For this review, take the finished solid that the model builds, in its own axes (mm). Give positions to 0.01 mm unless a question says otherwise; leave off trailing zeros. Order: outer loops, then holes, each group sorted by start corner. A loop starts at its lowest first (then second) coordinate and runs counter-clockwise, first axis right, second up.
from build123d import *

# Parameters (mm, degrees)
CROQUIS1_W              = 56
CROQUIS1_H              = 55
SALIENTE_EXTRUIR1_DEPTH = 3
CROQUIS2_R              = 1.3
CORTAR_EXTRUIR1_DEPTH   = 4
CROQUIS3_R              = 6.3
CROQUIS3_R_2            = 1.25
CORTAR_EXTRUIR2_DEPTH   = 4


with BuildPart() as part:
    # Croquis1 → Saliente-Extruir1 (new body)
    with BuildSketch(Plane.XY):
        with Locations((1.5, 0)):
            Rectangle(CROQUIS1_W, CROQUIS1_H)
    extrude(amount=SALIENTE_EXTRUIR1_DEPTH)

    # Croquis2 → Cortar-Extruir1 (cut)
    with BuildSketch(Plane.XY.offset(3)):
        with Locations((25.5, 23.528824725)):
            Circle(CROQUIS2_R)
        with Locations((19.5, 23.528824725)):
            Circle(CROQUIS2_R)
        with Locations((-22.5, 23.528824725)):
            Circle(CROQUIS2_R)
        with Locations((-16.5, 23.528824725)):
            Circle(CROQUIS2_R)
        with Locations((24.5, -14.75)):
            Circle(CROQUIS2_R)
    extrude(amount=-CORTAR_EXTRUIR1_DEPTH, mode=Mode.SUBTRACT)

    # Croquis3 → Cortar-Extruir2 (cut)
    with BuildSketch(Plane(origin=(0, 0, 0), x_dir=(-1, 0, 0), z_dir=(0, 0, -1))):
        with Locations((7, 8.5)):
            Circle(CROQUIS3_R)
        with Locations((20.6, 8.5)):
            Circle(CROQUIS3_R_2)
        with Locations((-6.1, 8.5)):
            Circle(CROQUIS3_R_2)
    extrude(amount=-CORTAR_EXTRUIR2_DEPTH, mode=Mode.SUBTRACT)


solid = part.part
1) Clearance check with a flat-ended pin moving along its axis: pin 1 (1.6 mm diameter, centred on x = -22.5, y = 23.53, fed in from +Z). State where the tip first meets the part, or that it passes through.
Answer sheet:
pin 1: passes through
2) Draft analysis for pull direction Y (two halves, no side actions). For faces 1 (the face through (-23.458, 24.407, 1.521)), 2 (the face through (1, 27.5, 1)), 3 (the face through (1, -27.5, 1)), 4 (the face through (1, 0, 0)), state which applies: +Y half, -Y half, draft (parallel to the pull), parting line (faces both ways), or undercut.
Answer sheet:
face 1: undercut
face 2: +Y half
face 3: -Y half
face 4: draft
3) We need section A-A on x = -22.5. Give the boundary of the cut face in (y, z).
Answer sheet:
outline: (-27.5, 0) - (22.23, 0) - (22.23, 3) - (-27.5, 3) - close; (24.83, 0) - (27.5, 0) - (27.5, 3) - (24.83, 3) - close
4) We need section B-B on y = 6.5. Give the boundary of the cut face in (x, z), then the cut area to 3 significant figures.
Answer sheet:
outline: (-26.5, 0) - (-12.97, 0) - (-12.97, 3) - (-26.5, 3) - close; (-1.03, 0) - (29.5, 0) - (29.5, 3) - (-1.03, 3) - close
area: 132 mm2
5) To check wall thickness, follow line 1 (Y direction, x = -7, z = 0.95); line 2 (Y direction, x = -16.5, z = 1.9); line 3 (Y direction, x = 24.5, z = 1.9). State the ranges of each line that lie inside material, in increasing order.
Answer sheet:
line 1: y = -27.5 to 2.2, 14.8 to 27.5
line 2: y = -27.5 to 22.23, 24.83 to 27.5
line 3: y = -27.5 to -16.05, -13.45 to 22.7, 24.36 to 27.5
6) We need section C-C on z = 1.9. Count the separate pieces of the cut face and the enclosed holes in it, then the cut area to 3 significant figures.
Answer sheet:
separate pieces: 1
enclosed holes: 8
area: 2,920 mm2
